from build123d import *

# Parameters (mm, degrees)
F1_DEPTH = 3.175
F2_W     = 27.94
F2_H     = 37.338
F2_W_2   = 3.302
F2_H_2   = 27.94
F3_DEPTH = 25.4


with BuildPart() as f1:
    # F0 (on Front) → F1 (new body)
    with BuildSketch(Plane.XZ):
        with BuildLine():
            ThreePointArc((152.4, 63.5), (148.680256, 72.480256), (139.7, 76.2))
            Line((139.7, 76.2), (-139.7, 76.2))
            ThreePointArc((-139.7, 76.2), (-148.680256, 72.480256), (-152.4, 63.5))
            Line((-152.4, 63.5), (-152.4, -63.5))
            ThreePointArc((-152.4, -63.5), (-148.680256, -72.480256), (-139.7, -76.2))
            Line((-139.7, -76.2), (139.7, -76.2))
            ThreePointArc((139.7, -76.2), (148.680256, -72.480256), (152.4, -63.5))
            Line((152.4, -63.5), (152.4, 63.5))
        make_face()
    extrude(amount=F1_DEPTH)

    # F2 (on face) → F3 (cut)
    with BuildSketch(Plane.XZ.offset(3.175)):
        with BuildLine():
            ThreePointArc((-144.78, -25.4), (-139.7, -30.48), (-134.62, -25.4))
            Line((-134.62, -25.4), (-134.62, 0))
            Line((-134.62, 0), (-134.62, 25.4))
            ThreePointArc((-134.62, 25.4), (-139.7, 30.48), (-144.78, 25.4))
            Line((-144.78, 25.4), (-144.78, 0))
            Line((-144.78, 0), (-144.78, -25.4))
        make_face()
        with BuildLine():
            ThreePointArc((55.88, 38.1), (50.8, 43.18), (45.72, 38.1))
            Line((45.72, 38.1), (45.72, 0))
            Line((45.72, 0), (45.72, -38.1))
            ThreePointArc((45.72, -38.1), (50.8, -43.18), (55.88, -38.1))
            Line((55.88, -38.1), (55.88, 0))
            Line((55.88, 0), (55.88, 38.1))
        make_face()
        with Locations((97.580589, 0)):
            Rectangle(F2_W, F2_H)
        with Locations((-139.7, 57.15)):
            Rectangle(F2_W_2, F2_H_2)
        with Locations((-139.7, -57.15)):
            Rectangle(F2_W_2, F2_H_2)
        with Locations((139.7, 57.15)):
            Rectangle(F2_W_2, F2_H_2)
        with Locations((139.7, -57.15)):
            Rectangle(F2_W_2, F2_H_2)
        with BuildLine():
            Line((134.62, 25.4), (134.62, 0))
            Line((134.62, 0), (134.62, -25.4))
            ThreePointArc((134.62, -25.4), (139.7, -30.48), (144.78, -25.4))
            Line((144.78, -25.4), (144.78, 0))
            Line((144.78, 0), (144.78, 25.4))
            ThreePointArc((144.78, 25.4), (139.7, 30.48), (134.62, 25.4))
        make_face()
        with BuildLine():
            ThreePointArc((-69.85, 38.1), (-76.2, 44.45), (-82.55, 38.1))
            Line((-82.55, 38.1), (-82.55, 0))
            Line((-82.55, 0), (-82.55, -38.1))
            ThreePointArc((-82.55, -38.1), (-76.2, -44.45), (-69.85, -38.1))
            Line((-69.85, -38.1), (-69.85, 0))
            Line((-69.85, 0), (-69.85, 38.1))
        make_face()
    extrude(amount=-F3_DEPTH, mode=Mode.SUBTRACT)


with BuildPart() as f4_1:
    # F4: copy of F1
    add(f1.part)


solid = f1.part
For this review, take the finished solid that the model builds, in its own axes (mm). A direction names the side the tool comes from. Round coordinates to 2 decimals unless told otherwise and drop trailing zeros. Write each loop counter-clockwise with the first axis right and the second up, starting at its lowest first coordinate (ties: lowest second). Pieces come first, ordered by that corner, then holes. Notation, with made-up numbers: (-26.75, 17) - (6.25, 17) arc R33 ccw to (6.25, 52) - close; hole circle Ø3 at (56.25, 17). An arc over 180 degrees is marked (long way). Use a Markdown table: item, result.
Q1. We need section B-B (z = -9). Give the boundary of the cut face in (x, y) (3 decimals), plus the area to 3 significant figures.
Derived:
| item | result |
|---|---|
| outline | (-152.4, -3.175) - (-144.78, -3.175) - (-144.78, 0) - (-152.4, 0) - close; (-134.62, -3.175) - (-82.55, -3.175) - (-82.55, 0) - (-134.62, 0) - close; (-69.85, -3.175) - (45.72, -3.175) - (45.72, 0) - (-69.85, 0) - close; (55.88, -3.175) - (83.611, -3.175) - (83.611, 0) - (55.88, 0) - close; (111.551, -3.175) - (134.62, -3.175) - (134.62, 0) - (111.551, 0) - close; (144.78, -3.175) - (152.4, -3.175) - (152.4, 0) - (144.78, 0) - close |
| area | 742 mm2 |
Q2. We need section A-A (x = -76.2). Give the boundary of the cut face in (y, z) (3 decimals), plus the area to 3 significant figures.
Derived:
| item | result |
|---|---|
| outline | (-3.175, -76.2) - (0, -76.2) - (0, -44.45) - (-3.175, -44.45) - close; (-3.175, 44.45) - (0, 44.45) - (0, 76.2) - (-3.175, 76.2) - close |
| area | 202 mm2 |
Q3. We need section D-D (y = -2.3). State how many separate pieces and enclosed holes the cut face has, plus the area to 3 significant figures.
Derived:
| item | result |
|---|---|
| separate pieces | 1 |
| enclosed holes | 9 |
| area | 41,800 mm2 |
Q4. The part is to be moulded in two halves that separate along X. For faces 3 (the cylindrical face through (-148.58, -1.57, 72.58)), 4 (the cylindrical face through (-76.34, -1.61, -44.45)), 5 (the flat face through (-2, 0, 1)), say which applies: pulls with the +X half, pulls with the -X half, needs draft (parallel to the pull), parting line crosses it, or undercut.
Derived:
| item | result |
|---|---|
| face 3 | pulls with the -X half |
| face 4 | undercut |
| face 5 | needs draft |
Q5. Machinability: for faces 1 (the cylindrical face through (-76.06, -1.61, 44.45)), 2 (the cylindrical face through (148.78, -1.57, 72.38)), which of the approach directions +Z, -Z, +X, -X, +Y, -Y give a long, thin tool a straight path to every point of the face, cutting with its end or side? Answer none if there is none.
Derived:
| item | result |
|---|---|
| face 1 | +Y, -Y |
| face 2 | +Z, +X, +Y, -Y |
Q6. Clearance check with flat-ended pins moving along their axes: pin 1 (1.6 mm diameter, centred on x = -140.5, y = -1.5, fed in from -Z); pin 2 (4 mm diameter, centred on x = 49.5, z = -11, fed in from +Y). State where each tip first meets the part, or that it passes through.
Derived:
| item | result |
|---|---|
| pin 1 | stops at z = -76.2 |
| pin 2 | passes through |
Q7. We need section C-C (z = 48). Give the boundary of the cut face in (x, y) (3 decimals), plus the area to 3 significant figures.
Derived:
| item | result |
|---|---|
| outline | (-152.4, -3.175) - (-141.351, -3.175) - (-141.351, 0) - (-152.4, 0) - close; (-138.049, -3.175) - (138.049, -3.175) - (138.049, 0) - (-138.049, 0) - close; (141.351, -3.175) - (152.4, -3.175) - (152.4, 0) - (141.351, 0) - close |
| area | 947 mm2 |
Q8. Wall thickness on line 1 along X through (y, z) = (-2.5, -37.5); line 2 along X through (y, z) = (-1.8, -58.5); line 3 along X through (y, z) = (-1.1, 10): over which ranges is each line inside the solid? List them lowest first.
Derived:
| item | result |
|---|---|
| line 1 | x = -152.4 to -82.55, -69.85 to 45.72, 55.88 to 152.4 |
| line 2 | x = -152.4 to -141.35, -138.05 to 138.05, 141.35 to 152.4 |
| line 3 | x = -152.4 to -144.78, -134.62 to -82.55, -69.85 to 45.72, 55.88 to 83.61, 111.55 to 134.62, 144.78 to 152.4 |
